The model under review builds one solid part; all positions refer to its coordinate system, in mm. A direction names the side the tool comes from. Round coordinates to 2 decimals unless told otherwise and drop trailing zeros. Loops run counter-clockwise (first coordinate to the right, second up) from the corner with the lowest first, then second, coordinate; pieces in that order, holes last. Notation, with made-up numbers: (-1, 86) -> (57, 86) arc R22 ccw to (57, 112) -> close; hole circle Ø2 at (-35, 65). An arc over 180 degrees is marked (long way). Return JSON: item names as keys, results as strings. Group by question number.
```python
from build123d import *

# Parameters (mm, degrees)
SKETCH_1_W          = 67
SKETCH_1_H          = 36
EXTRUDE_1_DEPTH     = 18
SKETCH_2_W          = 20
SKETCH_2_H          = 12
EXTRUDE_2_DEPTH     = 5
FILLET_1_R          = 8
SKETCH_3_R          = 2
CUT_EXTRUDE_1_DEPTH = 5


with BuildPart() as part:
    # 草图1 → 凸台-拉伸1 (new body)
    with BuildSketch(Plane(origin=(0, 0, 0), x_dir=(1, 0, 0), z_dir=(0, 1, 0))):
        Rectangle(SKETCH_1_W, SKETCH_1_H)
    extrude(amount=EXTRUDE_1_DEPTH)

    # 草图2 → 凸台-拉伸2 (add)
    with BuildSketch(Plane(origin=(0, 18, 0), x_dir=(1, 0, 0), z_dir=(0, 1, 0))):
        with Locations((23.5, 0)):
            Rectangle(SKETCH_2_W, SKETCH_2_H)
    extrude(amount=EXTRUDE_2_DEPTH)

    # 圆角1
    fillet_1_edges = [part.edges().sort_by_distance(p)[0] for p in [
        (0, 18, 18),
        (0, 0, 18),
        (0, 0, -18),
        (0, 18, -18),
    ]]
    fillet(fillet_1_edges, radius=FILLET_1_R)

    # 草图3 → 切除-拉伸1 (cut)
    with BuildSketch(Plane(origin=(33.5, 0, 0), x_dir=(0, 0, -1), z_dir=(1, 0, 0))):
        with Locations((2.5, 19.5)):
            Circle(SKETCH_3_R)
        with Locations((-2.3, 19.5)):
            Circle(SKETCH_3_R)
    extrude(amount=-CUT_EXTRUDE_1_DEPTH, mode=Mode.SUBTRACT)


solid = part.part
```
1. For P1, Ø1.5, axis at x = -2, y = 13.5, coming from the +Z side; P2, Ø12, axis at x = 17.5, y = 17, coming from the -Z side; P3, Ø2, axis at y = 20, z = 1.5, coming from the +X side, all flat-tipped, find the tip position at first contact; note any pin that passes through.
2. We need section D-D, the plane z = -1.5. Write out the cut boundary in (x, y).
3. We need section A-A, the plane z = 2.3. Write out the cut boundary in (x, y).
4. Wall thickness on line 1 (Y direction, x = 31.7, z = 2.3); line 2 (Y direction, x = -13, z = -6.5); line 3 (Y direction, x = 10, z = 15.5): over which ranges is each line inside the solid? List them lowest first.
5. We need section C-C, the plane y = 19.5. Write out the cut boundary in (x, z).
6. Tool access review of faces 1 (the face through (31.035, 21.483, 2.56)), 2 (the face through (13.5, 20, 0)), 3 (the face through (0, 0, 0)): name each direction out of +Z, -Z, +X, -X, +Y, -Y from which nothing blocks a thin tool from reaching the whole face with its end or side.
7. Draft analysis for pull direction Z (two halves, no side actions). For faces 4 (the face through (31.035, 21.483, -2.24)), 5 (the face through (23, 20, 6)), 6 (the face through (23, 20, -6)), 7 (the face through (28.5, 20, -2)), state which applies: pulls with the +Z half, pulls with the -Z half, needs draft (parallel to the pull), parting line crosses it, or undercut.
8. We need section B-B, the plane x = -10. Write out the cut boundary in (y, z), then the cut area to 3 significant figures.
Check sheet entries:
{
 "1": {"P1": "stops at z = 17.51", "P2": "stops at z = -17.94", "P3": "stops at x = 28.5"},
 "2": {"outline": "(-33.5, 0) -> (33.5, 0) -> (33.5, 17.77) -> (28.5, 17.77) -> (28.5, 21.23) -> (33.5, 21.23) -> (33.5, 23) -> (13.5, 23) -> (13.5, 18) -> (-33.5, 18) -> close"},
 "3": {"outline": "(-33.5, 0) -> (33.5, 0) -> (33.5, 17.5) -> (28.5, 17.5) -> (28.5, 21.5) -> (33.5, 21.5) -> (33.5, 23) -> (13.5, 23) -> (13.5, 18) -> (-33.5, 18) -> close"},
 "4": {"line 1": "y = 0 to 17.5, 21.5 to 23", "line 2": "y = 0 to 18", "line 3": "y = 2.19 to 15.81"},
 "5": {"outline": "(13.5, -6) -> (33.5, -6) -> (33.5, -4.5) -> (28.5, -4.5) -> (28.5, -0.5) -> (33.5, -0.5) -> (33.5, 0.3) -> (28.5, 0.3) -> (28.5, 4.3) -> (33.5, 4.3) -> (33.5, 6) -> (13.5, 6) -> close"},
 "6": {"face 1": "+X", "face 2": "+Z, -Z, -X, +Y", "face 3": "+Z, -Z, +X, -X, -Y"},
 "7": {"face 4": "undercut", "face 5": "pulls with the +Z half", "face 6": "pulls with the -Z half", "face 7": "undercut"},
 "8": {"outline": "(0, -10) arc R8 ccw to (8, -18) -> (10, -18) arc R8 ccw to (18, -10) -> (18, 10) arc R8 ccw to (10, 18) -> (8, 18) arc R8 ccw to (0, 10) -> close", "area": "593 mm²"}
}
